Input: part model. Units: mm. Frame: model coordinates. Face numbers are marked on the shaded views. A direction names the side the tool comes from. Round coordinates to 2 decimals unless told otherwise and drop trailing zeros. Write each loop counter-clockwise with the first axis right and the second up, starting at its lowest first coordinate (ties: lowest second). Pieces come first, ordered by that corner, then holes. Notation, with made-up numbers: (68.5, -33.75) - (82.5, -33.75) arc R21 ccw to (82.5, -6.75) - close; hole circle Ø8 at (87.5, 57.5). An arc over 180 degrees is marked (long way). Use one line per item in the form item = value.
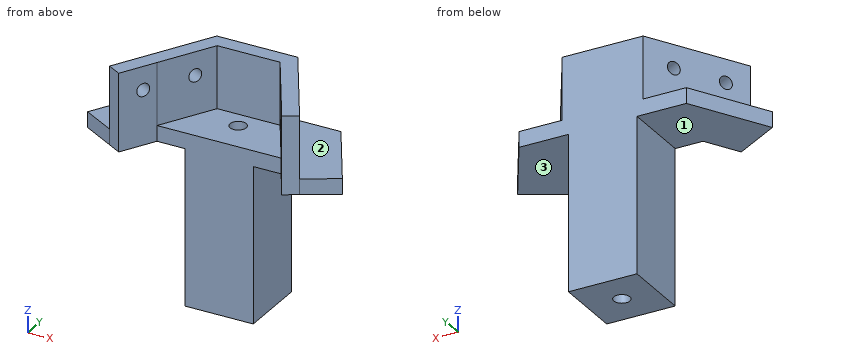
```python
from build123d import *

# Parameters (mm, degrees)
F1_DEPTH = 5
F2_DEPTH = 25
F4_D     = 4.2
F6_W     = 22
F6_H     = 22
F7_DEPTH = 50
F9_D     = 5.2


with BuildPart() as f1:
    # F0 (on Top) → F1 (new body)
    with BuildSketch(Plane.XY):
        Polygon((10.113249, -5), (0, -5), (0, -22), (19.928203, -22), align=None)
        Polygon((13, 0), (0, 0), (0, -5), (10.113249, -5), (19.928203, -22), (26.169873, -32.810889), (30.5, -30.310889), align=None)
        Polygon((26.856406, 0), (13, 0), (30.5, -30.310889), (40.892305, -24.310889), align=None)
    extrude(amount=F1_DEPTH)

    # F0 (on Top) → F2 (join)
    with BuildSketch(Plane.XY):
        Polygon((13, 0), (0, 0), (0, -5), (10.113249, -5), (19.928203, -22), (26.169873, -32.810889), (30.5, -30.310889), align=None)
    extrude(amount=F2_DEPTH)

    # F4 (through all)
    with Locations(Plane(origin=(9.75, 5.629165, 0), x_dir=(-0.5, 0.866025, 0), z_dir=(0.866025, 0.5, 0))):
        with Locations((-33.5, 17.5), (-16.5, 17.5)):
            Hole(F4_D / 2)

    # F5: F1 across plane


with BuildPart() as f1_1:
    add(f1.part)
    add(f1.part.mirror(Plane.YZ))

    # F6 (on face) → F7 (join)
    with BuildSketch(Plane(origin=(0, 0, 0), x_dir=(1, 0, 0), z_dir=(0, 0, -1))):
        with Locations((0, 11)):
            Rectangle(F6_W, F6_H)
    extrude(amount=F7_DEPTH)

    # F9 (through all)
    with Locations(Plane(origin=(0, 0, -50), x_dir=(1, 0, 0), z_dir=(0, 0, -1))):
        with Locations((0, 11)):
            Hole(F9_D / 2)


solid = f1_1.part
```
(1) Cut plane C-C on z = -20.5. Output: boundary loops of the cut face in (x, y).
Derived:
outline = (-11, -22) - (11, -22) - (11, 0) - (-11, 0) - close; hole circle Ø5.2 at (0, -11)
(2) Access query for the marked faces 1, 2 and 3. Directions: +Z, -Z, +X, -X, +Y, -Y. A direction counts if a zero-diameter tool reaches every point of the face in a straight line with its end or side. Return the directions, or none.
Derived:
face_1 = -Z, -X, +Y, -Y
face_2 = +Z, +X, +Y
face_3 = -Z, +X, +Y, -Y
(3) First-contact query: pin 1 Ø4 at (x, y) = (0, -11) entering from +Z; pin 2 Ø2 at (x, z) = (-8.5, -17.5) entering from -Y; pin 3 Ø8 at (y, z) = (-19.5, -9.5) entering from +X; pin 4 Ø10 at (y, z) = (-11, -34.5) entering from -X. Flat tips, straight axial feed; report the tip coordinate or a pass-through.
Derived:
pin_1 = through
pin_2 = -22
pin_3 = 11
pin_4 = -11
(4) Cut plane B-B on z = 10.5. Output: boundary loops of the cut face in (x, y).
Derived:
outline = (-30.5, -30.31) - (-26.17, -32.81) - (-10.11, -5) - (10.11, -5) - (26.17, -32.81) - (30.5, -30.31) - (13, 0) - (-13, 0) - close
(5) Material intervals for L1, parallel to Y at x = 0, z = -34; L2, parallel to X at y = -11, z = -9; L3, parallel to Z at x = 10, y = -14, sorted ascending.
Derived:
L1 = -22 to -13.6, -8.4 to 0
L2 = -11 to -2.6, 2.6 to 11
L3 = -50 to 5
(6) Cut plane D-D on y = -18. Output: boundary loops of the cut face in (x, z), then the cut area to 3 significant figures.
Derived:
outline = (-37.25, 0) - (-11, 0) - (-11, -50) - (11, -50) - (11, 0) - (37.25, 0) - (37.25, 5) - (23.39, 5) - (23.39, 25) - (17.62, 25) - (17.62, 5) - (-17.62, 5) - (-17.62, 25) - (-23.39, 25) - (-23.39, 5) - (-37.25, 5) - close
area = 1,700 mm^2
(7) Cut plane A-A on x = 0. Output: boundary loops of the cut face in (y, z), then the cut area to 3 significant figures.
Derived:
outline = (-22, -50) - (-13.6, -50) - (-13.6, 5) - (-22, 5) - close; (-8.4, -50) - (0, -50) - (0, 25) - (-5, 25) - (-5, 5) - (-8.4, 5) - close
area = 1,020 mm^2
